```python
from build123d import *

# Parameters (mm, degrees)
SKETCH_1_W          = 106
SKETCH_1_H          = 25
SKETCH_1_R          = 1.65
SKETCH_1_R_2        = 2.15
EXTRUDE_1_DEPTH     = 2
SKETCH_2_W          = 106
SKETCH_2_H          = 6
EXTRUDE_3_DEPTH     = 2
SKETCH_4_R          = 1.65
CUT_EXTRUDE_1_DEPTH = 57.171612047
CUT_EXTRUDE_2_DEPTH = 10
SKETCH_6_W          = 106
SKETCH_6_H          = 4
CUT_EXTRUDE_3_DEPTH = 57.171612047
FILLET_1_R          = 2


with BuildPart() as part:
    # 草图1 → 凸台-拉伸1 (new body)
    with BuildSketch(Plane.XY):
        Rectangle(SKETCH_1_W, SKETCH_1_H)
        with Locations((-28, 5.5)):
            Circle(SKETCH_1_R, mode=Mode.SUBTRACT)
        with Locations(Location((-28, -7.5, 0), (0, 0, 180))):
            Circle(SKETCH_1_R, mode=Mode.SUBTRACT)
        with Locations((28, -7.5)):
            Circle(SKETCH_1_R, mode=Mode.SUBTRACT)
        with Locations(Location((28, 5.5, 0), (0, 0, 180))):
            Circle(SKETCH_1_R, mode=Mode.SUBTRACT)
        with Locations((-48, 5.5)):
            Circle(SKETCH_1_R, mode=Mode.SUBTRACT)
        with Locations(Location((48, 5.5, 0), (0, 0, 180))):
            Circle(SKETCH_1_R, mode=Mode.SUBTRACT)
        with Locations((0, -5)):
            Circle(SKETCH_1_R_2, mode=Mode.SUBTRACT)
    extrude(amount=EXTRUDE_1_DEPTH)

    # 草图2 → 凸台-拉伸3 (add)
    with BuildSketch(Plane.XY.offset(2)):
        with Locations((0, -15.5)):
            Rectangle(SKETCH_2_W, SKETCH_2_H)
    extrude(amount=-EXTRUDE_3_DEPTH)

    # 草图4 → 切除-拉伸1 (cut, through all)
    with BuildSketch(Plane.XY.offset(2)):
        with Locations((-48, -15.5)):
            Circle(SKETCH_4_R)
        with Locations(Location((48, -15.5, 0), (0, 0, 180))):
            Circle(SKETCH_4_R)
        with Locations((-28, -15.5)):
            Circle(SKETCH_4_R)
        with Locations(Location((28, -15.5, 0), (0, 0, 180))):
            Circle(SKETCH_4_R)
    extrude(amount=-CUT_EXTRUDE_1_DEPTH, mode=Mode.SUBTRACT)

    # 草图5 → 切除-拉伸2 (cut)
    with BuildSketch(Plane.XY.offset(2)):
        with BuildLine():
            Line((-17.5, -3.35), (-7.5, -3.35))
            ThreePointArc((-7.5, -3.35), (-5.85, -5), (-7.5, -6.65))
            Line((-7.5, -6.65), (-17.5, -6.65))
            ThreePointArc((-17.5, -6.65), (-19.15, -5), (-17.5, -3.35))
        make_face()
        with BuildLine():
            Line((17.5, -3.35), (7.5, -3.35))
            ThreePointArc((7.5, -3.35), (5.85, -5), (7.5, -6.65))
            Line((7.5, -6.65), (17.5, -6.65))
            ThreePointArc((17.5, -6.65), (19.15, -5), (17.5, -3.35))
        make_face()
    extrude(amount=-CUT_EXTRUDE_2_DEPTH, mode=Mode.SUBTRACT)

    # 草图6 → 切除-拉伸3 (cut, through all)
    with BuildSketch(Plane.XY.offset(2)):
        with Locations((0, 10.5)):
            Rectangle(SKETCH_6_W, SKETCH_6_H)
    extrude(amount=-CUT_EXTRUDE_3_DEPTH, mode=Mode.SUBTRACT)

    # 圆角1
    fillet_1_edges = [part.edges().sort_by_distance(p)[0] for p in [
        (-53, 8.5, 1),
        (53, 8.5, 1),
        (-53, -18.5, 1),
        (53, -18.5, 1),
    ]]
    fillet(fillet_1_edges, radius=FILLET_1_R)


solid = part.part
```
Here's how the part is built. I have some questions about the finished solid (model axes, mm). A direction names the side the tool comes from. Coordinates: 2 decimals unless noted, no trailing zeros. Loops run counter-clockwise (first coordinate to the right, second up) from the corner with the lowest first, then second, coordinate; pieces in that order, holes last. Notation, with made-up numbers: (82.25, 5) - (94.25, 5) arc R4 ccw to (94.25, 10) - close; hole circle Ø10 at (5.5, 32). An arc over 180 degrees is marked (long way). Return JSON: item names as keys, results as strings. Group by question number.
Item 1: We'd pull the mould along X, two halves only. Please class faces 3 (the face through (-52.43, -17.9, 0.99)), 4 (the face through (53, -5, 1)), 5 (the face through (19.15, -5.04, 1.01)): +X half, -X half, draft (parallel to the pull), parting line (faces both ways), or undercut.
Item 2: If we section it at B-B on y = 5.5: Write out the boundary of the cut face in (x, z), and give its area (3 significant figures).
Item 3: If we section it at A-A on x = 28: Write out the boundary of the cut face in (y, z).
Item 4: If we section it at D-D on x = -48: Write out the boundary of the cut face in (y, z), and give its area (3 significant figures).
Item 5: On a 3-axis mill with a long thin cutter (end or side, diameter ignored), from which of +Z, -Z, +X, -X, +Y, -Y can I reach the whole of each face in a straight line? I mean faces 1 (the face through (-1, -2, 2)), 2 (the face through (-19.15, -5.04, 1.01)). Say none if no direction works.
Item 6: I need wall thicknesses on line 1 (Y direction, x = -48, z = 1.2); line 2 (Y direction, x = -28, z = 0.8); line 3 (Y direction, x = -13.5, z = 0.3). Which ranges of each line are inside material? Lowest first, please. Write a range as from..to.
Item 7: Will this pin go through, and if not, where does the flat tip stop? P1, Ø5.5, axis at x = -28, y = -15.5, coming from the +Z side.
Item 8: If we section it at C-C on z = 1.65: State how many separate pieces and enclosed holes the cut face has, and give its area (3 significant figures).
Calculated:
{
 "1": {"face 3": "-X half", "face 4": "+X half", "face 5": "undercut"},
 "2": {"outline": "(-53, 0) - (-49.65, 0) - (-49.65, 2) - (-53, 2) - close; (-46.35, 0) - (-29.65, 0) - (-29.65, 2) - (-46.35, 2) - close; (-26.35, 0) - (26.35, 0) - (26.35, 2) - (-26.35, 2) - close; (29.65, 0) - (46.35, 0) - (46.35, 2) - (29.65, 2) - close; (49.65, 0) - (53, 0) - (53, 2) - (49.65, 2) - close", "area": "186 mm^2"},
 "3": {"outline": "(-18.5, 0) - (-17.15, 0) - (-17.15, 2) - (-18.5, 2) - close; (-13.85, 0) - (-9.15, 0) - (-9.15, 2) - (-13.85, 2) - close; (-5.85, 0) - (3.85, 0) - (3.85, 2) - (-5.85, 2) - close; (7.15, 0) - (8.5, 0) - (8.5, 2) - (7.15, 2) - close"},
 "4": {"outline": "(-18.5, 0) - (-17.15, 0) - (-17.15, 2) - (-18.5, 2) - close; (-13.85, 0) - (3.85, 0) - (3.85, 2) - (-13.85, 2) - close; (7.15, 0) - (8.5, 0) - (8.5, 2) - (7.15, 2) - close", "area": "40.8 mm^2"},
 "5": {"face 1": "+Z, +X, -X, +Y, -Y", "face 2": "+Z, -Z"},
 "6": {"line 1": "y = -18.5..-17.15, -13.85..3.85, 7.15..8.5", "line 2": "y = -18.5..-17.15, -13.85..-9.15, -5.85..3.85, 7.15..8.5", "line 3": "y = -18.5..-6.65, -3.35..8.5"},
 "7": {"P1": "stops at z = 2"},
 "8": {"separate pieces": "1", "enclosed holes": "13", "area": "2,680 mm^2"}
}
